Model file for the job. Use its own axes, mm. A direction names the side the tool comes from. Give positions to 0.01 mm unless a question says otherwise; leave off trailing zeros. Write each loop counter-clockwise with the first axis right and the second up, starting at its lowest first coordinate (ties: lowest second). Pieces come first, ordered by that corner, then holes. Notation, with made-up numbers: (36.5, -31) - (54.5, -31) arc R22 cw to (54.5, 2) - close; hole circle Ø9 at (21, 49.5). An arc over 180 degrees is marked (long way). Use CSV: the item, a comma, the result in double quotes.
from build123d import *

# Parameters (mm, degrees)
SKETCH2_R                = 5.95
BOSS_EXTRUDE2_DEPTH      = 2.4
BOSS_EXTRUDE3_DEPTH      = 1.55
BOSS_EXTRUDE3_DEPTH_BACK = 1.55


with BuildPart() as part:
    # Sketch2 → Boss-Extrude2 (new body)
    with BuildSketch(Plane(origin=(0, 0, 0), x_dir=(1, 0, 0), z_dir=(0, 1, 0))):
        with Locations(Location((0, 0, 0), (0, 0, 270))):
            Circle(SKETCH2_R)
    extrude(amount=BOSS_EXTRUDE2_DEPTH)

    # Sketch4 → Boss-Extrude3 (add, two sides: drawn at the far end of the back side and taken through both)
    with BuildSketch(Plane.XY.offset(-BOSS_EXTRUDE3_DEPTH_BACK)):
        Polygon((-0.85, 2.4), (-0.85, 4.5), (-2.55, 4.5), (-2.55, 6.6), (2.55, 6.6), (2.55, 4.5), (0.85, 4.5), (0.85, 2.4), align=None)
    extrude(amount=BOSS_EXTRUDE3_DEPTH + BOSS_EXTRUDE3_DEPTH_BACK)


solid = part.part
(1) Saw through at A-A, the plane z = 0. List the corners of the cut face in (x, y), then the cut area to 3 significant figures.
Checked values:
outline,"(-5.95, 0) - (5.95, 0) - (5.95, 2.4) - (0.85, 2.4) - (0.85, 4.5) - (2.55, 4.5) - (2.55, 6.6) - (-2.55, 6.6) - (-2.55, 4.5) - (-0.85, 4.5) - (-0.85, 2.4) - (-5.95, 2.4) - close"
area,"42.8 mm^2"
(2) Saw through at B-B, the plane x = 0. List the corners of the cut face in (y, z), then the cut area to 3 significant figures.
Checked values:
outline,"(0, -5.95) - (2.4, -5.95) - (2.4, -1.55) - (6.6, -1.55) - (6.6, 1.55) - (2.4, 1.55) - (2.4, 5.95) - (0, 5.95) - close"
area,"41.6 mm^2"
(3) Saw through at D-D, the plane z = -1.25. List the corners of the cut face in (x, y), then the cut area to 3 significant figures.
Checked values:
outline,"(-5.82, 0) - (5.82, 0) - (5.82, 2.4) - (0.85, 2.4) - (0.85, 4.5) - (2.55, 4.5) - (2.55, 6.6) - (-2.55, 6.6) - (-2.55, 4.5) - (-0.85, 4.5) - (-0.85, 2.4) - (-5.82, 2.4) - close"
area,"42.2 mm^2"
(4) Flat gauge pins, fed straight in: P1, Ø1.5, axis at x = -2.5, y = 1, coming from the +Z side; P2, Ø2.5, axis at y = 6, z = 0, coming from the -X side; P3, Ø0.6, axis at y = 4, z = 0.5, coming from the -X side. Where does each tip first touch, or does it go through?
Checked values:
P1,"stops at z = 5.69"
P2,"stops at x = -2.55"
P3,"stops at x = -0.85"
(5) Pull direction Y, two halves, no side cores. Call faces 6 (the face through (0, 6.6, 0)), 7 (the face through (-0.85, 3, 0)), 8 (the face through (0, 5, 1.55)): released by +Y, released by -Y, zero draft, split by the parting line, or undercut.
Checked values:
face 6,"released by +Y"
face 7,"undercut"
face 8,"zero draft"
(6) Saw through at C-C, the plane y = 5.25. List the corners of the cut face in (x, z).
Checked values:
outline,"(-2.55, -1.55) - (2.55, -1.55) - (2.55, 1.55) - (-2.55, 1.55) - close"
(7) 3-axis set-ups, long thin cutter, end or side, ignore diameter. For faces 1 (the face through (2.55, 6, 0)), 2 (the face through (0, 5, -1.55)), 3 (the face through (0.85, 3, 0)), 4 (the face through (-2, 4.5, 0)), 5 (the face through (-2.55, 6, 0)): which of +Z, -Z, +X, -X, +Y, -Y reach the whole face in a straight line?
Checked values:
face 1,"+Z, -Z, +X, +Y"
face 2,"-Z, +X, -X, +Y"
face 3,"+Z, -Z, +X"
face 4,"+Z, -Z, -X"
face 5,"+Z, -Z, -X, +Y"
(8) Wall check: probe 1 along Y at (x, z) = (0, 4.75); probe 2 along X at (y, z) = (5, -1.25); probe 3 along Z at (x, y) = (0.5, 4). Give the ranges that are in metal, low to high. Write a range as [from, to].
Checked values:
probe 1,"y = [0, 2.4]"
probe 2,"x = [-2.55, 2.55]"
probe 3,"z = [-1.55, 1.55]"
